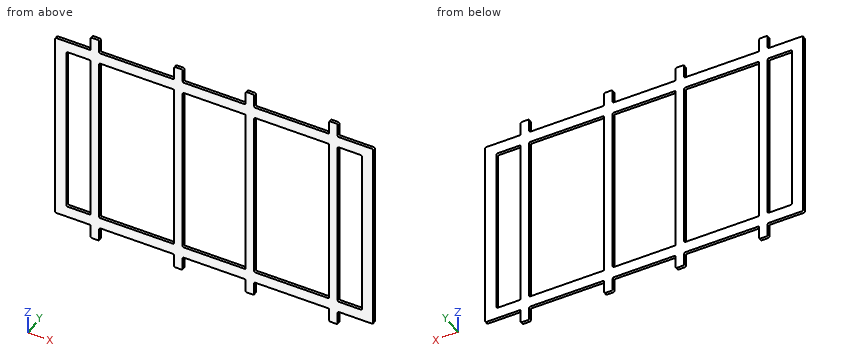
```python
from build123d import *

# Parameters (mm, degrees)
SKETCH1_W               = 560
SKETCH1_H               = 344
BOSS_EXTRUDE1_DEPTH     = 5
SKETCH2_W               = 15
SKETCH2_H               = 25
BOSS_EXTRUDE2_DEPTH     = 5
MIRROR5_COPY_1_SKETCH_W = 15
MIRROR5_COPY_1_SKETCH_H = 25
MIRROR5_COPY_1_DEPTH    = 5
FILLET3_R               = 2
SKETCH3_W               = 42.5
SKETCH3_H               = 304
SKETCH3_W_2             = 132
SKETCH3_W_3             = 55.5
CUT_EXTRUDE1_DEPTH      = 343.394509302
FILLET4_R               = 2


with BuildPart() as part:
    # Sketch1 → Boss-Extrude1 (new body)
    with BuildSketch(Plane(origin=(0, 0, 0), x_dir=(1, 0, 0), z_dir=(0, 1, 0))):
        Rectangle(SKETCH1_W, SKETCH1_H)
    extrude(amount=BOSS_EXTRUDE1_DEPTH)

    # Sketch2 → Boss-Extrude2 (add)
    with BuildSketch(Plane(origin=(0, 5, 0), x_dir=(1, 0, 0), z_dir=(0, 1, 0))):
        with Locations((-63, -184.5)):
            Rectangle(SKETCH2_W, SKETCH2_H)
        with Locations((-210, -184.5)):
            Rectangle(SKETCH2_W, SKETCH2_H)
    boss_extrude2 = extrude(amount=-BOSS_EXTRUDE2_DEPTH)

    # Mirror4: Boss-Extrude2 across plane
    add(boss_extrude2.mirror(Plane(origin=(0, 0, 0), x_dir=(0, 0, 1), z_dir=(1, 0, 0))))

    # Mirror5: Boss-Extrude2 across plane
    add(boss_extrude2.mirror(Plane.XY))

    # Mirror5 copy 1 sketch → Mirror5 copy 1 (add)
    with BuildSketch(Plane(origin=(0, 5, 0), x_dir=(-1, 0, 0), z_dir=(0, 1, 0))):
        with Locations((-63, -184.5)):
            Rectangle(MIRROR5_COPY_1_SKETCH_W, MIRROR5_COPY_1_SKETCH_H)
        with Locations((-210, -184.5)):
            Rectangle(MIRROR5_COPY_1_SKETCH_W, MIRROR5_COPY_1_SKETCH_H)
    extrude(amount=-MIRROR5_COPY_1_DEPTH)

    # Fillet3
    fillet3_edges = [part.edges().sort_by_distance(p)[0] for p in [
        (-70.5, 2.5, 197),
        (-70.5, 2.5, 172),
        (-55.5, 2.5, 172),
        (-55.5, 2.5, 197),
        (-202.5, 2.5, 172),
        (-202.5, 2.5, 197),
        (-217.5, 2.5, 197),
        (-217.5, 2.5, 172),
        (55.5, 2.5, 172),
        (55.5, 2.5, 197),
        (70.5, 2.5, 197),
        (70.5, 2.5, 172),
        (217.5, 2.5, 197),
        (217.5, 2.5, 172),
        (202.5, 2.5, 172),
        (202.5, 2.5, 197),
        (70.5, 2.5, -197),
        (70.5, 2.5, -172),
        (55.5, 2.5, -172),
        (55.5, 2.5, -197),
        (202.5, 2.5, -172),
        (202.5, 2.5, -197),
        (217.5, 2.5, -197),
        (217.5, 2.5, -172),
        (-280, 2.5, -172),
        (280, 2.5, -172),
        (280, 2.5, 172),
        (-280, 2.5, 172),
        (-55.5, 2.5, -172),
        (-55.5, 2.5, -197),
        (-70.5, 2.5, -197),
        (-70.5, 2.5, -172),
        (-217.5, 2.5, -197),
        (-217.5, 2.5, -172),
        (-202.5, 2.5, -172),
        (-202.5, 2.5, -197),
    ]]
    fillet(fillet3_edges, radius=FILLET3_R)

    # Sketch3 → Cut-Extrude1 (cut, through all)
    with BuildSketch(Plane(origin=(0, 5, 0), x_dir=(1, 0, 0), z_dir=(0, 1, 0))):
        with Locations((238.75, 0)):
            Rectangle(SKETCH3_W, SKETCH3_H)
        with Locations((136.5, 0)):
            Rectangle(SKETCH3_W_2, SKETCH3_H)
        with Locations((27.75, 0)):
            Rectangle(SKETCH3_W_3, SKETCH3_H)
    cut_extrude1 = extrude(amount=-CUT_EXTRUDE1_DEPTH, mode=Mode.SUBTRACT)

    # Mirror6: Cut-Extrude1 across plane
    add(cut_extrude1.mirror(Plane(origin=(0, 0, 0), x_dir=(0, 0, 1), z_dir=(1, 0, 0))), mode=Mode.SUBTRACT)

    # Fillet4
    fillet4_edges = [part.edges().sort_by_distance(p)[0] for p in [
        (217.5, 2.5, 152),
        (217.5, 2.5, -152),
        (260, 2.5, -152),
        (260, 2.5, 152),
        (202.5, 2.5, -152),
        (202.5, 2.5, 152),
        (70.5, 2.5, 152),
        (70.5, 2.5, -152),
        (55.5, 2.5, -152),
        (55.5, 2.5, 152),
        (-217.5, 2.5, -152),
        (-217.5, 2.5, 152),
        (-260, 2.5, 152),
        (-260, 2.5, -152),
        (-202.5, 2.5, 152),
        (-202.5, 2.5, -152),
        (-70.5, 2.5, -152),
        (-70.5, 2.5, 152),
        (-55.5, 2.5, 152),
        (-55.5, 2.5, -152),
    ]]
    fillet(fillet4_edges, radius=FILLET4_R)


solid = part.part
```
Model file for the job. Use its own axes, mm. Coordinates: 2 decimals unless noted, no trailing zeros. Order: outer loops, then holes, each group sorted by start corner. A loop starts at its lowest first (then second) coordinate and runs counter-clockwise, first axis right, second up. Notation, with made-up numbers: (-30, 13.5) - (-13, 13.5) arc R21 cw to (-13, 22.5) - close; hole circle Ø8 at (-21, 52). An arc over 180 degrees is marked (long way). Return JSON: item names as keys, results as strings. Group by question number.
1) Probe line 1 (X direction, y = 3.4, z = -64); line 2 (X direction, y = 3.9, z = -150.5); line 3 (Z direction, x = -138.5, y = 4). List the from-to ranges inside material, lowest first. Write a range as from..to.
2) Saw through at A-A, the plane z = -110.5. Write the cut outline in (x, y).
3) Saw through at C-C, the plane y = 1.95. Count the separate pieces of the cut face and the enclosed holes in it, plus the area to 3 significant figures.
4) Saw through at B-B, the plane x = -101.5. Write the cut outline in (y, z), plus the area to 3 significant figures.
5) Flat gauge pins, fed straight in: P1, Ø2, axis at x = 174, y = 1, coming from the +Z side; P2, Ø2.5, axis at x = 247, y = 2, coming from the -Z side; P3, Ø1.5, axis at y = 3.5, z = -189.5, coming from the -X side. Where does each tip first touch, or does it go through?
Values found:
{
 "1": {"line 1": "x = -280..-260, -217.5..-202.5, -70.5..-55.5, 55.5..70.5, 202.5..217.5, 260..280", "line 2": "x = -280..-259.94, -217.56..-202.44, -70.56..-55.44, 55.44..70.56, 202.44..217.56, 259.94..280", "line 3": "z = -172..-152, 152..172"},
 "2": {"outline": "(-280, 0) - (-260, 0) - (-260, 5) - (-280, 5) - close; (-217.5, 0) - (-202.5, 0) - (-202.5, 5) - (-217.5, 5) - close; (-70.5, 0) - (-55.5, 0) - (-55.5, 5) - (-70.5, 5) - close; (55.5, 0) - (70.5, 0) - (70.5, 5) - (55.5, 5) - close; (202.5, 0) - (217.5, 0) - (217.5, 5) - (202.5, 5) - close; (260, 0) - (280, 0) - (280, 5) - (260, 5) - close"},
 "3": {"separate pieces": "1", "enclosed holes": "5", "area": "55,800 mm²"},
 "4": {"outline": "(0, -172) - (5, -172) - (5, -152) - (0, -152) - close; (0, 152) - (5, 152) - (5, 172) - (0, 172) - close", "area": "200 mm²"},
 "5": {"P1": "stops at z = 172", "P2": "stops at z = -172", "P3": "stops at x = -217.5"}
}
